Build history of the part. All positions in model axes, mm. A direction names the side the tool comes from. Coordinates: 2 decimals unless noted, no trailing zeros. Loops run counter-clockwise (first coordinate to the right, second up) from the corner with the lowest first, then second, coordinate; pieces in that order, holes last.
Item 1: Flat gauge pins, fed straight in: pin 1 (0.9 mm diameter, centred on x = 7.5, z = 0.5, fed in from -Y); pin 2 (7.5 mm diameter, centred on x = 20.5, y = -2, fed in from -Z); pin 3 (7 mm diameter, centred on y = 0, z = 0, fed in from -X). Where does each tip first touch, or does it go through?
Item 2: Cut at A-A (z = 0). List the corners of the cut face in (x, y).
Item 3: Cut at D-D (y = 0). List the corners of the cut face in (x, z), and give its area (3 significant figures).
Item 4: Cut at B-B (y = -5). List the corners of the cut face in (x, z), and give its area (3 significant figures).
Item 5: 3-axis set-ups, long thin cutter, end or side, ignore diameter. For faces 5 (the face through (22.5, -1.3, 1.3)), 6 (the face through (21.5, -6.02, 0.07)), 7 (the face through (26.06, 0.01, -7.51)): which of +Z, -Z, +X, -X, +Y, -Y reach the whole face in a straight line?
Item 6: Mould opens along X. For faces 1 (the face through (23, -4.5, 0)), 2 (the face through (15, 0, -6.75)), 3 (the face through (6.5, -6.02, 0.07)), 4 (the face through (0, -3.4, 0.1)) say: released by +X, released by -X, zero draft, split by the parting line, or undercut.
Item 7: Drill centre lines: line 1 along Y through (x, z) = (3.75, 2.5); line 2 along Y through (x, z) = (10.75, 0); line 3 along Z through (x, y) = (8, -5.4). Where is each one in solid material? Low to high.
Item 8: Cut at C-C (x = 3.25). List the corners of the cut face in (y, z), and give its area (3 significant figures).
from build123d import *

# Parameters (mm, degrees)
SKETCH1_W           = 30
SKETCH1_H           = 15
BOSS_EXTRUDE1_DEPTH = 6.75
SKETCH3_R           = 1.5
CUT_EXTRUDE1_DEPTH  = 3
BOSS_EXTRUDE2_DEPTH = 2
FILLET1_R           = 1


with BuildPart() as part:
    # Sketch1 → Boss-Extrude1 (new body, symmetric)
    with BuildSketch(Plane.XY):
        with Locations((15, 0)):
            Rectangle(SKETCH1_W, SKETCH1_H)
    extrude(amount=BOSS_EXTRUDE1_DEPTH, both=True)

    # Sketch3 → Cut-Extrude1 (cut)
    with BuildSketch(Plane.XZ.offset(7.5)):
        with Locations((8, 0)):
            Circle(SKETCH3_R)
        with Locations((23, 0)):
            Circle(SKETCH3_R)
    extrude(amount=-CUT_EXTRUDE1_DEPTH, mode=Mode.SUBTRACT)

    # Sketch4 → Boss-Extrude2 (add, symmetric)
    with BuildSketch(Plane(origin=(0, 0, 0), x_dir=(1, 0, 0), z_dir=(0, 1, 0))):
        Polygon((30, 6.75), (30, 8.25), (22, 6.75), align=None)
    extrude(amount=BOSS_EXTRUDE2_DEPTH, both=True)

    # Fillet1
    fillet1_edges = [part.edges().sort_by_distance(p)[0] for p in [
        (26, -2, -7.5),
        (26, 2, -7.5),
    ]]
    fillet(fillet1_edges, radius=FILLET1_R)

    # Sketch2 → Cut-Revolve1 (revolve, cut)
    with BuildSketch(Plane(origin=(0, 0, 0), x_dir=(1, 0, 0), z_dir=(0, 1, 0))):
        Polygon((0, 0), (30, 0), (30, 1.65), (22.5, 1.65), (22.5, 3), (0, 3), align=None)
    revolve(axis=Axis((0, 0, 0), (1, 0, 0)), mode=Mode.SUBTRACT)


solid = part.part
Filled sheet:
1. pin 1: stops at y = -4.5
1. pin 2: stops at z = -7.15
1. pin 3: stops at x = 0
2. outline: (0, -7.5) - (6.5, -7.5) - (6.5, -4.5) - (9.5, -4.5) - (9.5, -7.5) - (21.5, -7.5) - (21.5, -4.5) - (24.5, -4.5) - (24.5, -7.5) - (30, -7.5) - (30, -1.65) - (22.5, -1.65) - (22.5, -3) - (0, -3) - close; (0, 3) - (22.5, 3) - (22.5, 1.65) - (30, 1.65) - (30, 7.5) - (0, 7.5) - close
3. outline: (0, -6.75) - (22, -6.75) - (30, -8.25) - (30, -1.65) - (22.5, -1.65) - (22.5, -3) - (0, -3) - close; (0, 3) - (22.5, 3) - (22.5, 1.65) - (30, 1.65) - (30, 6.75) - (0, 6.75) - close
3. area: 251 mm2
4. outline: (0, -6.75) - (30, -6.75) - (30, 6.75) - (0, 6.75) - close; hole circle Ø3 at (8, 0); hole circle Ø3 at (23, 0)
4. area: 391 mm2
5. face 5: -X
5. face 6: -Y
5. face 7: -Z, -X, +Y, -Y
6. face 1: undercut
6. face 2: zero draft
6. face 3: undercut
6. face 4: released by -X
7. line 1: y = -7.5 to -1.66, 1.66 to 7.5
7. line 2: y = -7.5 to -3, 3 to 7.5
7. line 3: z = -6.75 to -1.5, 1.5 to 6.75
8. outline: (-7.5, -6.75) - (7.5, -6.75) - (7.5, 6.75) - (-7.5, 6.75) - close; hole circle Ø6 at (0, 0)
8. area: 174 mm2
